Could you check a few things on this model? Use its own coordinates, in mm. Face numbers are marked on the shaded views. Give positions to 0.01 mm unless a question says otherwise; leave off trailing zeros. Loops run counter-clockwise (first coordinate to the right, second up) from the corner with the lowest first, then second, coordinate; pieces in that order, holes last. Notation, with made-up numbers: (-0.5, 79) -> (37.5, 79) arc R35 ccw to (37.5, 115) -> close; hole circle Ø10 at (77.25, 38). An arc over 180 degrees is marked (long way). Write item = value, one per line. Start each with the question number.
1) I want a section at D-D (z = 2). List the corners of the cut face in (x, y) for me, and give its area (3 significant figures).
2) If we mould it in two halves opening along Y, with no side actions, what happens to the marked faces 1, 2 and 3? For each: +Y half, -Y half, draft (parallel to the pull), parting line (faces both ways), or undercut.
3) I want a section at C-C (z = 5.85). List the corners of the cut face in (x, y) for me, and give its area (3 significant figures).
4) I want a section at B-B (y = 7.75). List the corners of the cut face in (x, z) for me.
5) I want a section at A-A (x = 11). List the corners of the cut face in (y, z) for me.
6) I'm going to push a flat-ended pin straight in: pin 1 Ø3 at (y, z) = (4, 4) entering from -X. Where does the tip first touch, or does it pass through?
7) I need wall thicknesses on probe 1 along Y at (x, z) = (4.25, 5.5); probe 2 along Y at (x, z) = (10.75, 1.75); probe 3 along Y at (x, z) = (5.75, 4). Which ranges of each line are inside material? Lowest first, please. Write a range as from..to.
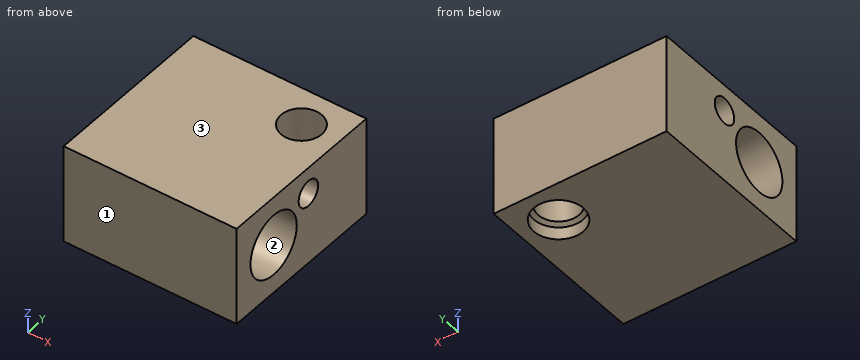
from build123d import *

# Parameters (mm, degrees)
SKETCH1_W                    = 14
SKETCH1_H                    = 14
BOSS_EXTRUDE1_DEPTH          = 8
M4X0_7_TAPPED_HOLE1_D        = 3.3
F_5_0_5_DIAMETER_HOLE1_D     = 5
F_2_1_2_1_DIAMETER_HOLE1_D   = 2.1
F_4_0_4_DIAMETER_HOLE1_D     = 4
F_4_0_4_DIAMETER_HOLE1_DEPTH = 1
F_4_0_4_DIAMETER_HOLE1_TIP   = 1.201721238


with BuildPart() as part:
    # Sketch1 → Boss-Extrude1 (new body)
    with BuildSketch(Plane.XY):
        with Locations((7, 7)):
            Rectangle(SKETCH1_W, SKETCH1_H)
    extrude(amount=BOSS_EXTRUDE1_DEPTH)

    # M4x0.7 Tapped Hole1 (through all)
    with Locations(Plane.XY.offset(8)):
        with Locations((11, 11)):
            Hole(M4X0_7_TAPPED_HOLE1_D / 2)

    # Ø5.0 (5) Diameter Hole1 (through all)
    with Locations(Plane.ZY):
        with Locations((4, 4)):
            Hole(F_5_0_5_DIAMETER_HOLE1_D / 2)

    # Ø2.1 (2.1) Diameter Hole1 (through all)
    with Locations(Plane.ZY):
        with Locations((5.85, 7.75)):
            Hole(F_2_1_2_1_DIAMETER_HOLE1_D / 2)

    # Ø4.0 (4) Diameter Hole1
    with Locations(Plane(origin=(11, 11, 0), x_dir=(-1, 0, 0), z_dir=(0, 0, -1))):
        with Locations((0, 0)):
            Hole(F_4_0_4_DIAMETER_HOLE1_D / 2, depth=F_4_0_4_DIAMETER_HOLE1_DEPTH)
            with Locations((0, 0, -(F_4_0_4_DIAMETER_HOLE1_DEPTH + F_4_0_4_DIAMETER_HOLE1_TIP / 2))):  # 118° drill point
                Cone(0, F_4_0_4_DIAMETER_HOLE1_D / 2, F_4_0_4_DIAMETER_HOLE1_TIP, mode=Mode.SUBTRACT)


solid = part.part
Answer list:
q1.outline = (0, 0) -> (14, 0) -> (14, 2.5) -> (0, 2.5) -> close; (0, 5.5) -> (14, 5.5) -> (14, 14) -> (0, 14) -> close; hole circle Ø3.3 at (11, 11)
q1.area = 145 mm^2
q2.face_1 = -Y half
q2.face_2 = undercut
q2.face_3 = draft
q3.outline = (0, 0) -> (14, 0) -> (14, 2.32) -> (0, 2.32) -> close; (0, 5.68) -> (14, 5.68) -> (14, 6.7) -> (0, 6.7) -> close; (0, 8.8) -> (14, 8.8) -> (14, 14) -> (0, 14) -> close; hole circle Ø3.3 at (11, 11)
q3.area = 111 mm^2
q4.outline = (0, 0) -> (14, 0) -> (14, 4.8) -> (0, 4.8) -> close; (0, 6.9) -> (14, 6.9) -> (14, 8) -> (0, 8) -> close
q5.outline = (0, 0) -> (9, 0) -> (9, 1) -> (9.35, 1.21) -> (9.35, 8) -> (0, 8) -> close; (12.65, 1.21) -> (13, 1) -> (13, 0) -> (14, 0) -> (14, 8) -> (12.65, 8) -> close; hole circle Ø5 at (4, 4); hole circle Ø2.1 at (7.75, 5.85)
q6.pin_1 = through
q7.probe_1 = 0..2, 6..6.76, 8.74..14
q7.probe_2 = 0..2.91, 5.09..9.37, 12.63..14
q7.probe_3 = 0..1.5, 6.5..14
